from build123d import *

# Parameters (mm, degrees)
SKETCH_1_R          = 5
SKETCH_1_R_2        = 3
EXTRUDE_1_DEPTH     = 5
SKETCH_2_R          = 10
SKETCH_2_R_2        = 3
EXTRUDE_2_DEPTH     = 2
SKETCH_3_R          = 5
EXTRUDE_3_DEPTH     = 3
SKETCH_4_R          = 10
EXTRUDE_4_DEPTH     = 2
SKETCH_5_R          = 3
CUT_EXTRUDE_1_DEPTH = 16.779733838
M3X0_5_1_REACH      = 22.665
M3X0_5_1_BORE_R     = 1.25


with BuildPart() as part:
    # ｽｹｯﾁ1 → ﾎﾞｽ - 押し出し1 (new body)
    with BuildSketch(Plane.XY):
        Circle(SKETCH_1_R)
        Circle(SKETCH_1_R_2, mode=Mode.SUBTRACT)
    extrude(amount=EXTRUDE_1_DEPTH)

    # ｽｹｯﾁ2 → ﾎﾞｽ - 押し出し2 (add)
    with BuildSketch(Plane.XY.offset(5)):
        Circle(SKETCH_2_R)
        Circle(SKETCH_2_R_2, mode=Mode.SUBTRACT)
    extrude(amount=EXTRUDE_2_DEPTH)

    # ｽｹｯﾁ3 → ﾎﾞｽ - 押し出し3 (add)
    with BuildSketch(Plane.XY.offset(7)):
        Circle(SKETCH_3_R)
    extrude(amount=EXTRUDE_3_DEPTH)

    # ｽｹｯﾁ4 → ﾎﾞｽ - 押し出し4 (add)
    with BuildSketch(Plane.XY.offset(10)):
        Circle(SKETCH_4_R)
    extrude(amount=EXTRUDE_4_DEPTH)

    # ｽｹｯﾁ5 → ｶｯﾄ - 押し出し1 (cut, through all)
    with BuildSketch(Plane(origin=(0, 0, 7), x_dir=(-1, 0, 0), z_dir=(0, 0, -1))):
        Circle(SKETCH_5_R)
    extrude(amount=-CUT_EXTRUDE_1_DEPTH, mode=Mode.SUBTRACT)

    # M3x0.5 ねじ穴1 bore (on position points) → M3x0.5 ねじ穴1 (cut, up to next)
    with BuildSketch(Plane(origin=(0.251235543, -4.993684081, 2.143915345), x_dir=(-0.998736816219, -0.050247108654, 0), z_dir=(0.050247108654, -0.998736816219, 0)), mode=Mode.PRIVATE) as m3x0_5_1_sk1:
        Circle(M3X0_5_1_BORE_R)
    m3x0_5_1_tool1 = extrude(m3x0_5_1_sk1.sketch, amount=-M3X0_5_1_REACH, mode=Mode.PRIVATE) & part.part
    add(m3x0_5_1_tool1.solids().sort_by_distance((0.251236, -4.993684, 2.143915))[0], mode=Mode.SUBTRACT)


solid = part.part
The model under review builds one solid part; all positions refer to its coordinate system, in mm. A direction names the side the tool comes from. Coordinates: 2 decimals unless noted, no trailing zeros. Loops run counter-clockwise (first coordinate to the right, second up) from the corner with the lowest first, then second, coordinate; pieces in that order, holes last. Notation, with made-up numbers: (55.5, -34.5) -> (105.5, -34.5) arc R22 cw to (105.5, -16.5) -> close; hole circle Ø9 at (-29.5, 70.5). An arc over 180 degrees is marked (long way). Use a Markdown table: item, result. Add a question column.
1. Add section C-C on x = -3.25. Write out the cut boundary in (y, z), plus the area to 3 significant figures.
2. To check wall thickness, follow line 1 (Z direction, x = -2, y = 8); line 2 (Y direction, x = 0, z = 8.75); line 3 (X direction, y = -1.5, z = 4). State the ranges of each line that lie inside material, in increasing order.
3. Clearance check with flat-ended pins moving along their axes: pin 1 Ø9.5 at (x, y) = (0, 0) entering from -Z; pin 2 Ø1 at (y, z) = (-4.5, 6.5) entering from +X; pin 3 Ø3 at (x, y) = (-6, -4) entering from -Z; pin 4 Ø2 at (x, z) = (1.5, 5.5) entering from -Y. State where each tip first meets the part, or that it passes through.
4. Add section D-D on y = 0. Write out the cut boundary in (x, z), plus the area to 3 significant figures.
5. Machinability: for faces 1 (the face through (2.307, -4.436, 2.465)), 2 (the face through (-5, -2, 10)), 3 (the face through (-2.17, -9.76, 10.99)), which of the approach directions +Z, -Z, +X, -X, +Y, -Y give a long, thin tool a straight path to every point of the face, cutting with its end or side? Answer none if there is none.
6. Add section B-B on x = -5.5. Write out the cut boundary in (y, z), plus the area to 3 significant figures.
7. Draft analysis for pull direction Z (two halves, no side actions). For faces 4 (the face through (-1.08, -4.88, 8.48)), 5 (the face through (-0.1, -3.3, 0)), 6 (the face through (2.1, 2.4, 12)), 7 (the face through (-5, -2, 7)), state which applies: pulls with the +Z half, pulls with the -Z half, needs draft (parallel to the pull), parting line crosses it, or undercut.
8. Add section A-A on y = 6.25. Write out the cut boundary in (x, z).
Returned:
| question | item | result |
|---|---|---|
| 1 | outline | (-9.46, 5) -> (-3.8, 5) -> (-3.8, 0) -> (3.8, 0) -> (3.8, 5) -> (9.46, 5) -> (9.46, 7) -> (3.8, 7) -> (3.8, 10) -> (9.46, 10) -> (9.46, 12) -> (-9.46, 12) -> (-9.46, 10) -> (-3.8, 10) -> (-3.8, 7) -> (-9.46, 7) -> close |
| 1 | area | 136 mm² |
| 2 | line 1 | z = 5 to 7, 10 to 12 |
| 2 | line 2 | y = -5 to -3, 3 to 5 |
| 2 | line 3 | x = -4.77 to -2.6, 2.6 to 4.77 |
| 3 | pin 1 | stops at z = 0 |
| 3 | pin 2 | stops at x = 9.17 |
| 3 | pin 3 | stops at z = 5 |
| 3 | pin 4 | stops at y = -9.99 |
| 4 | outline | (-10, 5) -> (-5, 5) -> (-5, 0) -> (-3, 0) -> (-3, 12) -> (-10, 12) -> (-10, 10) -> (-5, 10) -> (-5, 7) -> (-10, 7) -> close; (3, 0) -> (5, 0) -> (5, 5) -> (10, 5) -> (10, 7) -> (5, 7) -> (5, 10) -> (10, 10) -> (10, 12) -> (3, 12) -> close |
| 4 | area | 88.0 mm² |
| 5 | face 1 | -Z |
| 5 | face 2 | none |
| 5 | face 3 | +Z, -Z |
| 6 | outline | (-8.35, 5) -> (8.35, 5) -> (8.35, 7) -> (-8.35, 7) -> close; (-8.35, 10) -> (8.35, 10) -> (8.35, 12) -> (-8.35, 12) -> close |
| 6 | area | 66.8 mm² |
| 7 | face 4 | undercut |
| 7 | face 5 | pulls with the -Z half |
| 7 | face 6 | pulls with the +Z half |
| 7 | face 7 | undercut |
| 8 | outline | (-7.81, 5) -> (7.81, 5) -> (7.81, 7) -> (-7.81, 7) -> close; (-7.81, 10) -> (7.81, 10) -> (7.81, 12) -> (-7.81, 12) -> close |
